from build123d import *

# Parameters (mm, degrees)
ESTRUSIONE_ESTRUSIONE1_DEPTH = 1.5


with BuildPart() as part:
    # Schizzo1 → Estrusione-Estrusione1 (new body, symmetric)
    with BuildSketch(Plane.XY):
        Polygon((25, 17.5), (28, 17.5), (28, 11.166666667), (25, 11.166666667), (25, 4.833333333), (28, 4.833333333), (28, -1.5), (25, -1.5), (25, -7.833333333), (28, -7.833333333), (28, -14.166666667), (25, -14.166666667), (25, -20.5), (17.857142857, -20.5), (17.857142857, -17.5), (10.714285714, -17.5), (10.714285714, -20.5), (3.571428571, -20.5), (3.571428571, -17.5), (-3.571428571, -17.5), (-3.571428571, -20.5), (-10.714285714, -20.5), (-10.714285714, -17.5), (-17.857142857, -17.5), (-17.857142857, -20.5), (-25, -20.5), (-25, -14.166666667), (-28, -14.166666667), (-28, -7.833333333), (-25, -7.833333333), (-25, -1.5), (-28, -1.5), (-28, 4.833333333), (-25, 4.833333333), (-25, 11.166666667), (-28, 11.166666667), (-28, 17.5), (-25, 17.5), align=None)
        with BuildLine():
            Line((-10, 14.5), (10, 14.5))
            ThreePointArc((10, 14.5), (14.5, 10), (10, 5.5))
            Line((10, 5.5), (-10, 5.5))
            ThreePointArc((-10, 5.5), (-14.5, 10), (-10, 14.5))
        make_face(mode=Mode.SUBTRACT)
    extrude(amount=ESTRUSIONE_ESTRUSIONE1_DEPTH, both=True)


solid = part.part
Work out the finished part from the listing and answer in its coordinate system (mm). A direction names the side the tool comes from. Coordinates: 2 decimals unless noted, no trailing zeros. Loops run counter-clockwise (first coordinate to the right, second up) from the corner with the lowest first, then second, coordinate; pieces in that order, holes last. Notation, with made-up numbers: (13, 74) -> (36, 74) arc R20 ccw to (36, 93) -> close; hole circle Ø8 at (20.5, 16). An arc over 180 degrees is marked (long way). Write each question's results on one line, items separated by ' | '. Start each with the question number.
1) Find section A-A on x = 7. Determine the outline of the cut face in (y, z), then the cut area to 3 significant figures.
2) Flat-ended cylindrical pins translate along their axes: P1, Ø0.9, axis at x = -26, z = 0, coming from the -Y side; P2, Ø1, axis at y = 5.5, z = 1, coming from the -X side; P3, Ø1.5, axis at y = -19.5, z = 0.5, coming from the +X side. Find the tip coordinate at first contact, or state that the pin passes through.
3) Consider line 1 along X through (y, z) = (-19, -0.45); line 2 along Y through (x, z) = (-9, 0.6); line 3 along Y through (x, z) = (-3, 0.85). Determine where each line is inside the solid, lowest interval first.
4) For faces 1 (the cylindrical face through (-14.5, 9.9, 0)), 2 (the flat face through (27, -1.5, 0)), 3 (the flat face through (-27, 4.833, 0)), determine the directions among +Z, -Z, +X, -X, +Y, -Y from which every point of the face is accessible in a straight line to the end or side of a thin tool.
5) Find section C-C on y = -4.5. Determine the outline of the cut face in (x, z).
6) Find section B-B on y = 10. Determine the outline of the cut face in (x, z).
7) The mould has two halves that part along X. Classify faces 4 (the flat face through (-3.571, -19, 0)), 5 (the flat face through (0, -1, 1.5)), 6 (the flat face through (28, 14, 0)): pulls with the +X half, pulls with the -X half, needs draft (parallel to the pull), parting line crosses it, or undercut.
Response values:
1) outline: (-20.5, -1.5) -> (5.5, -1.5) -> (5.5, 1.5) -> (-20.5, 1.5) -> close; (14.5, -1.5) -> (17.5, -1.5) -> (17.5, 1.5) -> (14.5, 1.5) -> close | area: 87.0 mm^2
2) P1: stops at y = -14.17 | P2: stops at x = -25 | P3: stops at x = 25
3) line 1: x = -25 to -17.86, -10.71 to -3.57, 3.57 to 10.71, 17.86 to 25 | line 2: y = -20.5 to 5.5, 14.5 to 17.5 | line 3: y = -17.5 to 5.5, 14.5 to 17.5
4) face 1: +Z, -Z | face 2: +Z, -Z, +X | face 3: +Z, -Z, -X
5) outline: (-25, -1.5) -> (25, -1.5) -> (25, 1.5) -> (-25, 1.5) -> close
6) outline: (-25, -1.5) -> (-14.5, -1.5) -> (-14.5, 1.5) -> (-25, 1.5) -> close; (14.5, -1.5) -> (25, -1.5) -> (25, 1.5) -> (14.5, 1.5) -> close
7) face 4: undercut | face 5: needs draft | face 6: pulls with the +X half
